Geometry check sheet. Reference: the model listing, model coordinates, mm. A direction names the side the tool comes from. Coordinates: 2 decimals unless noted, no trailing zeros. Order: outer loops, then holes, each group sorted by start corner. A loop starts at its lowest first (then second) coordinate and runs counter-clockwise, first axis right, second up. Notation, with made-up numbers: (-28.5, 26.25) - (8.5, 26.25) arc R18 cw to (8.5, 30.25) - close; hole circle Ø2 at (53, 24.5). An arc over 180 degrees is marked (long way). Put each result on its own line as item: value.
from build123d import *

# Parameters (mm, degrees)
FILLET1_R   = 0.25
FILLET2_R   = 0.3
HEX_2_DEPTH = 3


with BuildPart() as part:
    # BodySke → Base-Revolve (revolve)
    with BuildSketch(Plane.XY, mode=Mode.PRIVATE) as base_revolve_sk:
        Polygon((0, 0), (0, 5), (6, 5), (6, 3), (45.4455, 3), (46, 2.4455), (46, 0), align=None)
    revolve(base_revolve_sk.sketch.rotate(Axis((-31.75, 0, 0), (1, 0, 0)), 90), axis=Axis((-31.75, 0, 0), (1, 0, 0)))

    # Fillet1
    fillet1_edges = [part.edges().sort_by_distance(p)[0] for p in [
        (6, 0, -3),
    ]]
    fillet(fillet1_edges, radius=FILLET1_R)

    # Fillet2
    fillet2_edges = [part.edges().sort_by_distance(p)[0] for p in [
        (0, 0, -5),
    ]]
    fillet(fillet2_edges, radius=FILLET2_R)

    # Sketch2 → Hex-PreBroach (revolve, cut)
    with BuildSketch(Plane.XY, mode=Mode.PRIVATE) as hex_prebroach_sk:
        Polygon((0, 2.542), (3, 2.542), (4.467624384, 0), (0, 0), align=None)
    revolve(hex_prebroach_sk.sketch.rotate(Axis((0, 0, 0), (1, 0, 0)), 90), axis=Axis((0, 0, 0), (1, 0, 0)), mode=Mode.SUBTRACT)

    # Sketch3 → Hex 2 (cut)
    with BuildSketch(Plane(origin=(0, 0, 0), x_dir=(0, 0.500000000000001, 0.866025403784438), z_dir=(-1, 0, 0))):
        Polygon((1.467624384, 2.542), (-1.467624384, 2.542), (-2.935248769, 0), (-1.467624384, -2.542), (1.467624384, -2.542), (2.935248769, 0), align=None)
    extrude(amount=-HEX_2_DEPTH, mode=Mode.SUBTRACT)

    # Esquisse3 → Enlèvement de matière-Révolution1 (revolve, cut)
    with BuildSketch(Plane.XY, mode=Mode.PRIVATE) as enl_vement_de_mati_re_r_volution1_sk:
        with BuildLine():
            Line((43.4, 0), (46, 0))
            Line((46, 0), (46, -1.907878403))
            ThreePointArc((46, -1.907878403), (44.216784043, -1.61245155), (43.4, 0))
        make_face()
    revolve(enl_vement_de_mati_re_r_volution1_sk.sketch.rotate(Axis((43.4, 0, 0), (1, 0, 0)), 90), axis=Axis((43.4, 0, 0), (1, 0, 0)), mode=Mode.SUBTRACT)


solid = part.part
Q1. Depth check by flat-ended pin: pin 1 Ø5 at (x, y) = (13, -3.5) entering from +Z; pin 2 Ø0.6 at (y, z) = (-1.5, -1.5) entering from -X; pin 3 Ø5 at (x, y) = (41, -3.5) entering from -Z. Enter the tip coordinate at first touch or a pass-through.
Answer block:
pin 1: stops at z = 2.83
pin 2: stops at x = 3.07
pin 3: stops at z = -2.83
Q2. Thickness scan on L1, parallel to X at y = 4, z = -0.75; L2, parallel to Y at x = 36, z = 1.75; L3, parallel to Y at x = 24.5, z = 0. Record the ranges inside material, lowest first. Write a range as [from, to].
Answer block:
L1: x = [0, 6]
L2: y = [-2.44, 2.44]
L3: y = [-3, 3]
Q3. Access from +Z, -Z, +X, -X, +Y, -Y to the whole of each face (thin tool, end or side, straight path). Record for faces 1 (the flat face through (1.48, 2.19, 1.29)), 2 (the flat face through (6, 1, 3.3)), 3 (the flat face through (46, 2, -1)).
Answer block:
face 1: -X
face 2: +X
face 3: +Z, -Z, +X, +Y, -Y
Q4. Draft check along Z on faces 4 (the flat face through (0, 2, -2)), 5 (the flat face through (3, 1.4, -2.3)), 6 (the cylindrical face through (26.12, -0.9, 2.86)). Enter one of: pulls with the +Z half, pulls with the -Z half, needs draft (parallel to the pull), parting line crosses it, or undercut.
Answer block:
face 4: needs draft
face 5: undercut
face 6: parting line crosses it
Q5. Section check A-A on x = 18. Record the boundary of the cut face in (y, z).
Answer block:
outline: circle Ø6 at (0, 0)
